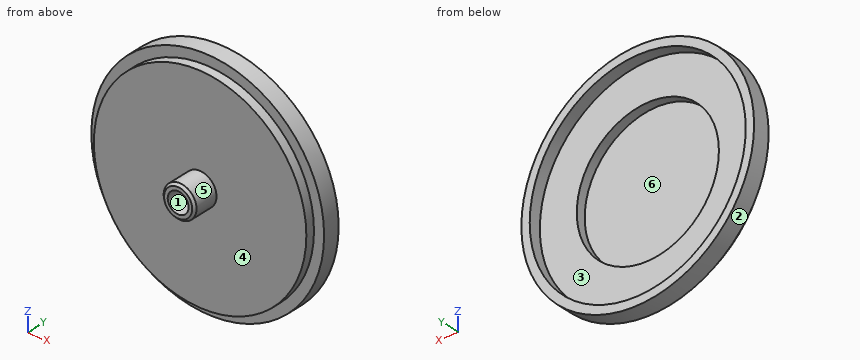
from build123d import *

# Parameters (mm, degrees)
F0_R      = 39.7
F1_DEPTH  = 5.9
F2_R      = 36.25
F3_DEPTH  = 3.1
F4_R      = 5.6
F5_DEPTH  = 8.9
F6_R      = 36.85
F7_DEPTH  = 4.1
F8_R      = 24.25
F9_DEPTH  = 3.2
F10_R     = 3.55
F11_DEPTH = 7.5
F12_SIZE  = 0.8


with BuildPart() as f1:
    # F0 (on Front) → F1 (new body)
    with BuildSketch(Plane.XZ):
        Circle(F0_R)
    extrude(amount=F1_DEPTH)

    # F2 (on face) → F3 (join)
    with BuildSketch(Plane.XZ.offset(5.9)):
        Circle(F2_R)
    extrude(amount=F3_DEPTH)

    # F4 (on face) → F5 (join)
    with BuildSketch(Plane.XZ.offset(9)):
        Circle(F4_R)
    extrude(amount=F5_DEPTH)

    # F6 (on face) → F7 (cut)
    with BuildSketch(Plane(origin=(0, 0, 0), x_dir=(-1, 0, 0), z_dir=(0, 1, 0))):
        Circle(F6_R)
    extrude(amount=-F7_DEPTH, mode=Mode.SUBTRACT)

    # F8 (on face) → F9 (cut)
    with BuildSketch(Plane(origin=(0, -4.1, 0), x_dir=(-1, 0, 0), z_dir=(0, 1, 0))):
        Circle(F8_R)
    extrude(amount=-F9_DEPTH, mode=Mode.SUBTRACT)

    # F10 (on face) → F11 (cut)
    with BuildSketch(Plane.XZ.offset(17.9)):
        Circle(F10_R)
    extrude(amount=-F11_DEPTH, mode=Mode.SUBTRACT)

    # F12
    f12_edges = [f1.edges().sort_by_distance(p)[0] for p in [
        (-5.6, -17.9, 0),
    ]]
    chamfer(f12_edges, length=F12_SIZE)


solid = f1.part
CAD build for the part. Positions are in the model's coordinates, mm. Face numbers are marked on the shaded views. A direction names the side the tool comes from. Give positions to 0.01 mm unless a question says otherwise; leave off trailing zeros. Loops run counter-clockwise (first coordinate to the right, second up) from the corner with the lowest first, then second, coordinate; pieces in that order, holes last. Notation, with made-up numbers: M 86,-33 L 90,-33 A11 cw 90,-27 Z; hole C 64,11.25 d4. An arc over 180 degrees is marked long. Answer in a Markdown table with one row per item. Add a question column.
Item 1: Probe probe 1 along Z at (x, y) = (0, -5.75); probe 2 along Y at (x, z) = (13.5, 30); probe 3 along X at (y, z) = (-4.5, 11). List the from-to ranges inside material, lowest first.
Item 2: Tool access for the marked faces 1, 2 and 3: list every direction of +Z, -Z, +X, -X, +Y, -Y with a clear straight run to the whole face (end or side of a thin tool).
Item 3: Band-saw the part on B-B on y = -14.75. Give the cut face in (x, z), then the cut area to 3 significant figures.
Item 4: Band-saw the part on D-D on z = -28. Give the cut face in (x, y), then the cut area to 3 significant figures.
Item 5: Mould opens along X. For the marked faces 4, 5 and 6 say: +X half, -X half, draft (parallel to the pull), parting line (faces both ways), or undercut.
Item 6: Band-saw the part on C-C on z = 0. Give the cut face in (x, y).
Item 7: Drop flat-ended pins along their axis: P1, Ø8, axis at y = -14, z = -5, coming from the -X side; P2, Ø4, axis at x = -30.5, z = 5, coming from the -Y side; P3, Ø6.5, axis at x = 0, z = 0, coming from the +Y side; P4, Ø8, axis at x = 24.5, z = -24, coming from the +Y side. Give the stop position or say it passes through.
Item 8: Band-saw the part on A-A on x = 0. Give the cut face in (y, z), then the cut area to 3 significant figures.
Reply:
| question | item | result |
|---|---|---|
| 1 | probe 1 | z = -39.7 to -24.25, 24.25 to 39.7 |
| 1 | probe 2 | y = -9 to -4.1 |
| 1 | probe 3 | x = -38.15 to -21.61, 21.61 to 38.15 |
| 2 | face 1 | -Y |
| 2 | face 2 | +Y, -Y |
| 2 | face 3 | +Y |
| 3 | outline | C 0,0 d11.2; hole C 0,0 d7.1 |
| 3 | area | 58.9 mm^2 |
| 4 | outline | M -28.14,-5.9 L -23.02,-5.9 L -23.02,-9 L 23.02,-9 L 23.02,-5.9 L 28.14,-5.9 L 28.14,0 L 23.96,0 L 23.96,-4.1 L -23.96,-4.1 L -23.96,0 L -28.14,0 Z |
| 4 | area | 278 mm^2 |
| 5 | face 4 | draft |
| 5 | face 5 | parting line |
| 5 | face 6 | undercut |
| 6 | outline | M -39.7,-5.9 L -36.25,-5.9 L -36.25,-9 L -5.6,-9 L -5.6,-17.1 L -4.8,-17.9 L -3.55,-17.9 L -3.55,-10.4 L 3.55,-10.4 L 3.55,-17.9 L 4.8,-17.9 L 5.6,-17.1 L 5.6,-9 L 36.25,-9 L 36.25,-5.9 L 39.7,-5.9 L 39.7,0 L 36.85,0 L 36.85,-4.1 L 24.25,-4.1 L 24.25,-7.3 L -24.25,-7.3 L -24.25,-4.1 L -36.85,-4.1 L -36.85,0 L -39.7,0 Z |
| 7 | P1 | stops at x = -5.51 |
| 7 | P2 | stops at y = -9 |
| 7 | P3 | stops at y = -7.3 |
| 7 | P4 | stops at y = 0 |
| 8 | outline | M -17.9,-4.8 L -17.1,-5.6 L -9,-5.6 L -9,-36.25 L -5.9,-36.25 L -5.9,-39.7 L 0,-39.7 L 0,-36.85 L -4.1,-36.85 L -4.1,-24.25 L -7.3,-24.25 L -7.3,24.25 L -4.1,24.25 L -4.1,36.85 L 0,36.85 L 0,39.7 L -5.9,39.7 L -5.9,36.25 L -9,36.25 L -9,5.6 L -17.1,5.6 L -17.9,4.8 L -17.9,3.55 L -10.4,3.55 L -10.4,-3.55 L -17.9,-3.55 Z |
| 8 | area | 282 mm^2 |
